Answer from the drawing. Dimensions are ordinates in mm from the lowest x, y and z of the part. Coordinates: 2 decimals unless noted, no trailing zeros. Write each loop counter-clockwise with the first axis right and the second up, starting at its lowest first coordinate (ties: lowest second). Pieces come first, ordered by that corner, then holes. Notation, with made-up numbers: (-5, 75) -> (20, 75) arc R9 ccw to (20, 85) -> close; hole circle Ø8 at (79.5, 12). An arc over 180 degrees is marked (long way). Return JSON: item names as keys, results as strings.
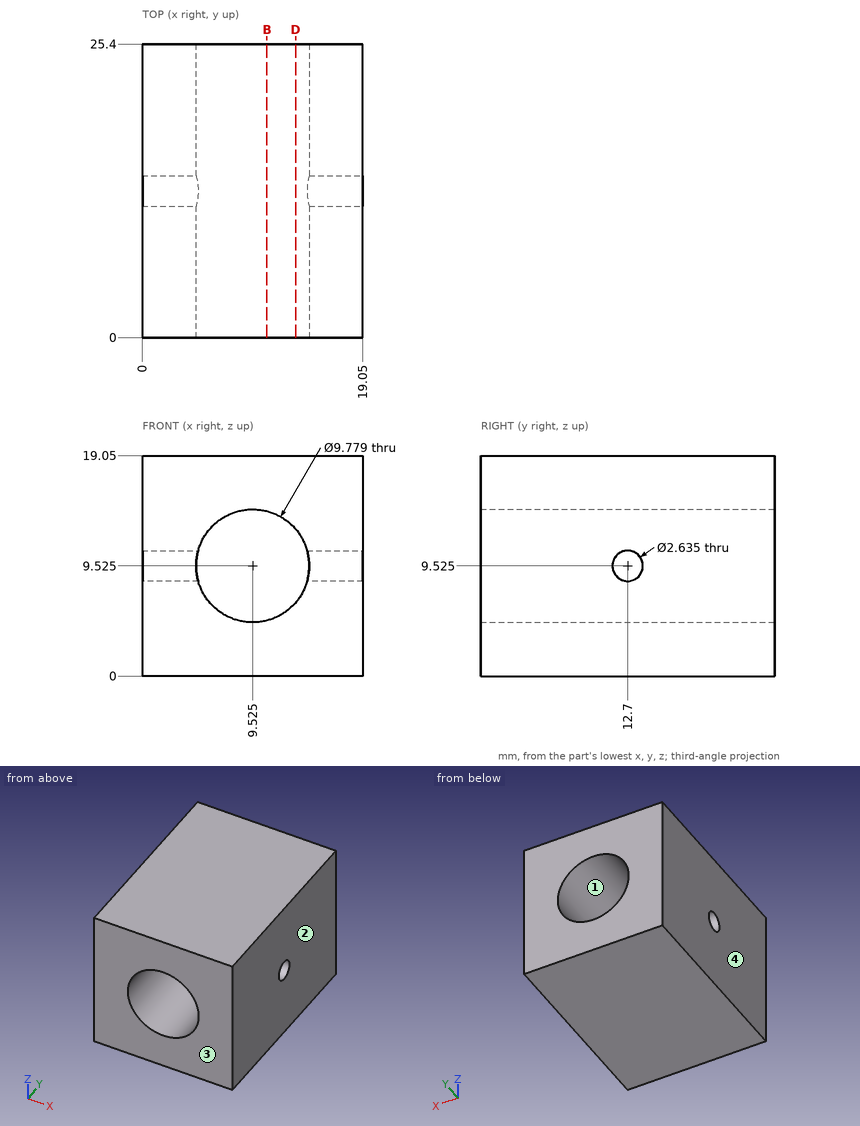
1. A flat-ended cylindrical pin translates along its axis: pin 1 Ø1.5 at (x, y) = (4, 3.5) entering from -Z. Find the tip coordinate at first contact, or state that the pin passes through.
Taken from the geometry:
{"pin 1": "stops at z = 0"}
2. For a pull along X with two mould halves and no side action, classify the marked faces 1, 2, 3 and 4 as +X half, -X half, draft (parallel to the pull), parting line (faces both ways), or undercut.
Taken from the geometry:
{"face 1": "undercut", "face 2": "+X half", "face 3": "draft", "face 4": "-X half"}
3. The part is cut by section B-B (x = 10.75). Determine the outline of the cut face in (y, z), then the cut area to 3 significant figures.
Taken from the geometry:
{"outline": "(0, 0) -> (25.4, 0) -> (25.4, 4.79) -> (0, 4.79) -> close; (0, 14.26) -> (25.4, 14.26) -> (25.4, 19.05) -> (0, 19.05) -> close", "area": "243 mm2"}
4. The part is cut by section D-D (x = 13.25). Determine the outline of the cut face in (y, z), then the cut area to 3 significant figures.
Taken from the geometry:
{"outline": "(0, 0) -> (25.4, 0) -> (25.4, 6.36) -> (0, 6.36) -> close; (0, 12.69) -> (25.4, 12.69) -> (25.4, 19.05) -> (0, 19.05) -> close", "area": "323 mm2"}
5. Consider L1, parallel to X at y = 15.25, z = 9.5; L2, parallel to X at y = 17.75, z = 8.5; L3, parallel to Z at x = 6, y = 18.25. Determine where each line is inside the solid, lowest interval first.
Taken from the geometry:
{"L1": "x = 0 to 4.64, 14.41 to 19.05", "L2": "x = 0 to 4.74, 14.31 to 19.05", "L3": "z = 0 to 6.14, 12.91 to 19.05"}
